The model under review builds one solid part; all positions refer to its coordinate system, in mm. Face numbers are marked on the shaded views. A direction names the side the tool comes from. Coordinates: 2 decimals unless noted, no trailing zeros. Write each loop counter-clockwise with the first axis right and the second up, starting at its lowest first coordinate (ties: lowest second). Pieces come first, ordered by that corner, then holes. Notation, with made-up numbers: (67, -1) -> (121, -1) arc R27 ccw to (121, 15) -> close; hole circle Ø11 at (60.5, 76.25). An arc over 180 degrees is marked (long way). Write each question's results on one line, items separated by ' | '.
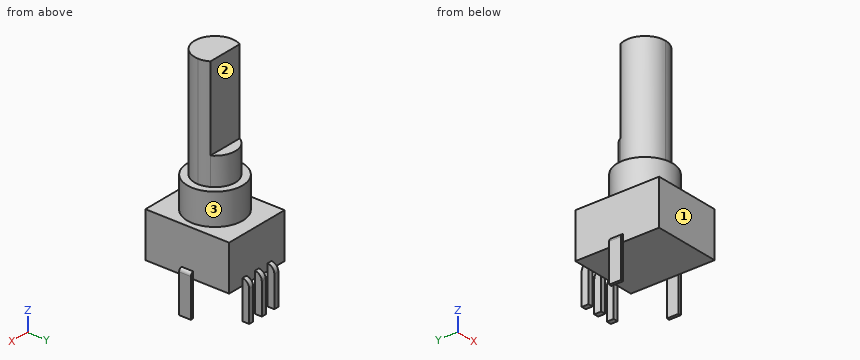
```python
from build123d import *

# Parameters (mm, degrees)
F0_W         = 9.7
F0_H         = 12.1
F0_R         = 4
F1_DEPTH     = 6.5
F2_DEPTH     = 4.5
F4_DEPTH     = 16
F5_DEPTH     = 4
F6_W         = 0.7
F6_H         = 4.5
F6_H_2       = 1
F6_W_2       = 0.35
F7_DEPTH     = 1
F8_R         = 0.99999
F9_W         = 0.85
F9_H         = 1
F10_DEPTH    = 0.4
F11_T1_DEPTH = 4.1494897428
F12_W        = 0.85
F12_H        = 1
F13_DEPTH    = 0.4
F14_T1_DEPTH = 4.1494897428


# Not quite as in the source:
# - a fillet or chamfer that OpenCascade refuses, or shapes differently, is made with other operations: its cross-section is extruded or revolved along the edge and cut away or added
# - a fillet or chamfer is up to 0.001 mm smaller than in the source, because OpenCascade refuses the exact size


with BuildPart() as f1:
    # F0 (on Top) → F1 (new body)
    with BuildSketch(Plane.XY):
        with Locations((-29.8902173527, 8.9015606931)):
            Rectangle(F0_W, F0_H)
        with Locations((-29.8902173527, 8.9015606931)):
            Circle(F0_R, mode=Mode.SUBTRACT)
        with Locations((-29.8902173527, 8.9015606931)):
            Circle(F0_R)
    extrude(amount=-F1_DEPTH)

    # F0 (on Top) → F2 (join)
    with BuildSketch(Plane.XY):
        with Locations((-29.8902173527, 8.9015606931)):
            Circle(F0_R)
    extrude(amount=F2_DEPTH)

    # F3 (on face) → F4 (join)
    with BuildSketch(Plane.XY.offset(4.5)):
        with BuildLine():
            ThreePointArc((-32.4592638684, 10.3515606931), (-32.4377651932, 7.4141132151), (-29.8902173527, 5.9515606931))
            Line((-29.8902173527, 5.9515606931), (-29.8902173527, 10.3515606931))
            Line((-29.8902173527, 10.3515606931), (-32.4592638684, 10.3515606931))
        make_face()
        with BuildLine():
            ThreePointArc((-29.8902173527, 5.9515606931), (-27.8042523482, 6.8155956886), (-26.9402173527, 8.9015606931))
            ThreePointArc((-26.9402173527, 8.9015606931), (-27.0370448008, 9.6511648482), (-27.3211708369, 10.3515606931))
            Line((-27.3211708369, 10.3515606931), (-29.8902173527, 10.3515606931))
            Line((-29.8902173527, 10.3515606931), (-29.8902173527, 5.9515606931))
        make_face()
    extrude(amount=F4_DEPTH)

    # F3 (on face) → F5 (join)
    with BuildSketch(Plane.XY.offset(4.5)):
        with BuildLine():
            Line((-29.8902173527, 10.3515606931), (-27.3211708369, 10.3515606931))
            ThreePointArc((-27.3211708369, 10.3515606931), (-29.8902173527, 11.8515606931), (-32.4592638684, 10.3515606931))
            Line((-32.4592638684, 10.3515606931), (-29.8902173527, 10.3515606931))
        make_face()
    extrude(amount=F5_DEPTH)

    # F6 (on face) → F7 (join)
    with BuildSketch(Plane(origin=(0, 14.9515606931, 0), x_dir=(-1, 0, 0), z_dir=(0, 1, 0))):
        with Locations((27.6902173527, -8.75)):
            Rectangle(F6_W, F6_H)
        with Locations((27.6902173527, -6)):
            Rectangle(F6_W, F6_H_2)
        with Locations((29.7152173527, -6)):
            Rectangle(F6_W_2, F6_H_2)
        with Locations((30.0652173527, -6)):
            Rectangle(F6_W_2, F6_H_2)
        Polygon((30.2402173527, -11), (30.2402173527, -6.5), (29.8902173527, -6.5), (29.5402173527, -6.5), (29.5402173527, -11), align=None)
        with Locations((32.0902173527, -6)):
            Rectangle(F6_W, F6_H_2)
        with Locations((32.0902173527, -8.75)):
            Rectangle(F6_W, F6_H)
    extrude(amount=F7_DEPTH)

    # F8 (radius 1 in the source; OpenCascade refuses exactly that, so slightly less here)
    f8_edges = [f1.edges().sort_by_distance(p)[0] for p in [
        (-27.690217, 15.951561, -5.5),
        (-29.890217, 15.951561, -5.5),
        (-32.090217, 15.951561, -5.5),
    ]]
    fillet(f8_edges, radius=F8_R)

    # F9 (on face) → F10 (join)
    with BuildSketch(Plane.YZ.offset(-25.0402173527)):
        with Locations((8.4765606931, -6)):
            Rectangle(F9_W, F9_H)
        with Locations((9.3265606931, -6)):
            Rectangle(F9_W, F9_H)
        Polygon((9.7515606931, -6.5), (8.9015606931, -6.5), (8.0515606931, -6.5), (8.0515606931, -11.5), (9.7515606931, -11.5), align=None)
    extrude(amount=F10_DEPTH)

    # F11: fillet of radius 0.5 on 1 edges, made by hand

    # F11_s2 → F11_t1 (cut)
    with BuildSketch(Plane.XZ.offset(-10.9763055645)):
        with BuildLine():
            ThreePointArc((-25.0402173527, -5.5), (-24.752919018, -5.6736701825), (-24.6402173527, -5.9898979486))
            Line((-24.6402173527, -5.9898979486), (-24.6402173527, -5.5))
            Line((-24.6402173527, -5.5), (-25.0402173527, -5.5))
        make_face()
    extrude(amount=F11_T1_DEPTH, mode=Mode.SUBTRACT)

    # F12 (on face) → F13 (join)
    with BuildSketch(Plane(origin=(-34.7402173527, 0, 0), x_dir=(0, -1, 0), z_dir=(-1, 0, 0))):
        with Locations((-9.3265606931, -6)):
            Rectangle(F12_W, F12_H)
        with Locations((-8.4765606931, -6)):
            Rectangle(F12_W, F12_H)
        Polygon((-8.9015606931, -6.5), (-9.7515606931, -6.5), (-9.7515606931, -11.5), (-8.0515606931, -11.5), (-8.0515606931, -6.5), align=None)
    extrude(amount=F13_DEPTH)

    # F14: fillet of radius 0.5 on 1 edges, made by hand

    # F14_s2 → F14_t1 (cut)
    with BuildSketch(Plane.XZ.offset(-10.9763055645)):
        with BuildLine():
            ThreePointArc((-34.7402173527, -5.5), (-35.0275156873, -5.6736701825), (-35.1402173527, -5.9898979486))
            Line((-35.1402173527, -5.9898979486), (-35.1402173527, -5.5))
            Line((-35.1402173527, -5.5), (-34.7402173527, -5.5))
        make_face()
    extrude(amount=F14_T1_DEPTH, mode=Mode.SUBTRACT)


solid = f1.part
```
Q1. Add section B-B (x = -33.5). Write out the cut boundary in (y, z).
Solution:
outline: (2.85, -6.5) -> (14.95, -6.5) -> (14.95, 0) -> (10.62, 0) -> (10.62, 4.5) -> (7.18, 4.5) -> (7.18, 0) -> (2.85, 0) -> close
Q2. For line 1 (Z direction, x = -31.25, y = 14); line 2 (Y direction, x = -31.75, z = -2.5); line 3 (Z direction, x = -26.75, y = 8.5), list the stretches that pass through material, from the lowest coordinate up. Write a range as from..to.
Solution:
line 1: -6.5..0 | line 2: 2.85..14.95 | line 3: -6.5..4.5
Q3. Clearance check with flat-ended pins moving along their axes: P1, Ø0.5, axis at y = 15.5, z = -8, coming from the +X side; P2, Ø1, axis at y = 4.5, z = 14.5, coming from the +X side; P3, Ø2, axis at x = -30.5, y = 5, coming from the -Z side; P4, Ø1.5, axis at x = -26.5, z = 3.5, coming from the +Y side. State where each tip first meets the part, or that it passes through.
Solution:
P1: x = -27.34 | P2: through | P3: z = -6.5 | P4: y = 11.91
Q4. Add section A-A (z = -7.5). Write out the cut boundary in (x, y), plus the area to 3 significant figures.
Solution:
outline: (-35.14, 8.05) -> (-34.74, 8.05) -> (-34.74, 9.75) -> (-35.14, 9.75) -> close; (-32.44, 14.95) -> (-31.74, 14.95) -> (-31.74, 15.95) -> (-32.44, 15.95) -> close; (-30.24, 14.95) -> (-29.54, 14.95) -> (-29.54, 15.95) -> (-30.24, 15.95) -> close; (-28.04, 14.95) -> (-27.34, 14.95) -> (-27.34, 15.95) -> (-28.04, 15.95) -> close; (-25.04, 8.05) -> (-24.64, 8.05) -> (-24.64, 9.75) -> (-25.04, 9.75) -> close | area: 3.46 mm²
Q5. Add section D-D (z = 1.5). Write out the cut boundary in (x, y), plus the area to 3 significant figures.
Solution:
outline: circle Ø8 at (-29.89, 8.9) | area: 50.3 mm²
Q6. Machinability: for the marked faces 1, 2 and 3, which of the approach directions +Z, -Z, +X, -X, +Y, -Y give a long, thin tool a straight path to every point of the face, cutting with its end or side? Answer none if there is none.
Solution:
face 1: +Z, -Z, +X, -X, -Y | face 2: +Z, +X, -X, +Y | face 3: +Z
Q7. Add section C-C (y = 4.5). Write out the cut boundary in (x, z).
Solution:
outline: (-34.74, -6.5) -> (-25.04, -6.5) -> (-25.04, 0) -> (-34.74, 0) -> close
